Input: part model. Units: mm. Frame: model coordinates. A direction names the side the tool comes from. Round coordinates to 2 decimals unless told otherwise and drop trailing zeros. Loops run counter-clockwise (first coordinate to the right, second up) from the corner with the lowest first, then second, coordinate; pieces in that order, holes last. Notation, with made-up numbers: M 53,54.25 L 68,54.25 A20 ccw 68,69.25 Z; hole C 56.25,-34 d9. An arc over 180 degrees is marked long. Use one line per item in the form item = value. Start each with the question number.
Q1. Ray query, line 1 along Z through (x, y) = (14, 8.89); line 2 along X through (y, z) = (11.5, 48.5); line 3 along Y through (x, z) = (-9, 15). Return the intervals inside material, ascending.
Q2. Section query B-B, the plane x = 0. Output: boundary loops of the cut face in (y, z).
Q3. Mould query, pull axis Y, two halves, no side actions, for faces 1 (the flat face through (-15.006, 6, 25)), 2 (the flat face through (14, 0, 25)), 3 (the cylindrical face through (-14.201, 11.264, 13.448)). Classes: pulls with the +Y half, pulls with the -Y half, needs draft (parallel to the pull), parting line crosses it, or undercut.
Q4. Section query A-A, the plane z = 38.1. Output: boundary loops of the cut face in (x, y).
Q5. Section query D-D, the plane z = 16. Output: boundary loops of the cut face in (x, y).
Q6. Section query C-C, the plane y = 15.25. Output: boundary loops of the cut face in (x, z).
Q7. First-contact query: P1, Ø8, axis at y = 8.89, z = 12.7, coming from the -X side; P2, Ø6, axis at x = -7.5, y = 14, coming from the +Z side. Flat tips, straight axial feed; report the tip coordinate or a pass-through.
Q8. Access query for faces 4 (the cylindrical face through (14.3, 18.38, 25.04)), 5 (the flat face through (3, 17.462, 25)). Directions: +Z, -Z, +X, -X, +Y, -Y. A direction counts if a zero-diameter tool reaches every point of the face in a straight line with its end or side. Return the directions, or none.
```python
from build123d import *

# Parameters (mm, degrees)
BASE_FLANGE1_DEPTH = 50.8
SKETCH6_R          = 2.4892
CUT_EXTRUDE1_DEPTH = 63.002427854
SKETCH7_R          = 2.4892
CUT_EXTRUDE2_DEPTH = 57.291492607


# Sheet-metal steps are written as plain solids
with BuildPart() as part:
    # Sketch1 → Base-Flange1 (new body)
    with BuildSketch(Plane.XY):
        with BuildLine():
            Line((-15.00632, 0), (-15.00632, 16.7005))
            ThreePointArc((-15.00632, 16.7005), (-14.318167382, 18.361847382), (-12.65682, 19.05))
            Line((-12.65682, 19.05), (12.65682, 19.05))
            ThreePointArc((12.65682, 19.05), (14.318167382, 18.361847382), (15.00632, 16.7005))
            Line((15.00632, 16.7005), (15.00632, 0))
            Line((15.00632, 0), (13.41882, 0))
            Line((13.41882, 0), (13.41882, 16.7005))
            ThreePointArc((13.41882, 16.7005), (13.195635367, 17.239315367), (12.65682, 17.4625))
            Line((12.65682, 17.4625), (-12.65682, 17.4625))
            ThreePointArc((-12.65682, 17.4625), (-13.195635367, 17.239315367), (-13.41882, 16.7005))
            Line((-13.41882, 16.7005), (-13.41882, 0))
            Line((-13.41882, 0), (-15.00632, 0))
        make_face()
    extrude(amount=BASE_FLANGE1_DEPTH)

    # Sketch6 → Cut-Extrude1 (cut, through all)
    with BuildSketch(Plane(origin=(15.00632, 0, 0), x_dir=(0, 0, -1), z_dir=(1, 0, 0))):
        with Locations(Location((-25.4, 8.89, 0), (0, 0, 90))):
            Circle(SKETCH6_R)
        with Locations(Location((-38.1, 8.89, 0), (0, 0, 90))):
            Circle(SKETCH6_R)
        with Locations(Location((-12.7, 8.89, 0), (0, 0, 90))):
            Circle(SKETCH6_R)
    extrude(amount=-CUT_EXTRUDE1_DEPTH, mode=Mode.SUBTRACT)

    # Sketch7 → Cut-Extrude2 (cut, through all)
    with BuildSketch(Plane(origin=(0, 19.05, 0), x_dir=(1, 0, 0), z_dir=(0, 1, 0))):
        with Locations(Location((0, -12.7, 0), (0, 0, 180))):
            Circle(SKETCH7_R)
        with Locations(Location((0, -25.4, 0), (0, 0, 180))):
            Circle(SKETCH7_R)
        with Locations(Location((0, -38.1, 0), (0, 0, 180))):
            Circle(SKETCH7_R)
    extrude(amount=-CUT_EXTRUDE2_DEPTH, mode=Mode.SUBTRACT)


solid = part.part
```
Results found:
q1.line_1 = 0 to 10.21, 15.19 to 22.91, 27.89 to 35.61, 40.59 to 50.8
q1.line_2 = -15.01 to -13.42, 13.42 to 15.01
q1.line_3 = 17.46 to 19.05
q2.outline = M 17.46,0 L 19.05,0 L 19.05,10.21 L 17.46,10.21 Z; M 17.46,15.19 L 19.05,15.19 L 19.05,22.91 L 17.46,22.91 Z; M 17.46,27.89 L 19.05,27.89 L 19.05,35.61 L 17.46,35.61 Z; M 17.46,40.59 L 19.05,40.59 L 19.05,50.8 L 17.46,50.8 Z
q3.face_1 = needs draft
q3.face_2 = pulls with the -Y half
q3.face_3 = undercut
q4.outline = M -15.01,0 L -13.42,0 L -13.42,6.4 L -15.01,6.4 Z; M -15.01,11.38 L -13.42,11.38 L -13.42,16.7 A0.76 cw -12.66,17.46 L -2.49,17.46 L -2.49,19.05 L -12.66,19.05 A2.35 ccw -15.01,16.7 Z; M 2.49,17.46 L 12.66,17.46 A0.76 cw 13.42,16.7 L 13.42,11.38 L 15.01,11.38 L 15.01,16.7 A2.35 ccw 12.66,19.05 L 2.49,19.05 Z; M 13.42,0 L 15.01,0 L 15.01,6.4 L 13.42,6.4 Z
q5.outline = M -15.01,0 L -13.42,0 L -13.42,16.7 A0.76 cw -12.66,17.46 L 12.66,17.46 A0.76 cw 13.42,16.7 L 13.42,0 L 15.01,0 L 15.01,16.7 A2.35 ccw 12.66,19.05 L -12.66,19.05 A2.35 ccw -15.01,16.7 Z
q6.outline = M -15.01,0 L -13.42,0 L -13.42,50.8 L -15.01,50.8 Z; M 13.42,0 L 15.01,0 L 15.01,50.8 L 13.42,50.8 Z
q7.P1 = -15.01
q7.P2 = through
q8.face_4 = +Z, -Z, +X, +Y
q8.face_5 = +Z, -Z, -Y
